```python
from build123d import *

# Parameters (mm, degrees)
SKETCH1_W           = 60
SKETCH1_H           = 52
SKETCH1_R           = 2.9
SKETCH1_R_2         = 3.05
BOSS_EXTRUDE1_DEPTH = 35
SKETCH2_R           = 5.5
CUT_EXTRUDE1_DEPTH  = 7
CHAMFER1_SIZE       = 0.4


with BuildPart() as part:
    # Sketch1 → Boss-Extrude1 (new body)
    with BuildSketch(Plane(origin=(0, 0, 0), x_dir=(1, 0, 0), z_dir=(0, 1, 0))):
        Rectangle(SKETCH1_W, SKETCH1_H)
        with Locations((-23, 6.5)):
            Circle(SKETCH1_R, mode=Mode.SUBTRACT)
        with Locations((23, 6.5)):
            Circle(SKETCH1_R, mode=Mode.SUBTRACT)
        with Locations((23, -6.5)):
            Circle(SKETCH1_R, mode=Mode.SUBTRACT)
        with Locations((-23, -6.5)):
            Circle(SKETCH1_R, mode=Mode.SUBTRACT)
        with Locations((-15, 18.5)):
            Circle(SKETCH1_R_2, mode=Mode.SUBTRACT)
        with Locations((15, 18.5)):
            Circle(SKETCH1_R_2, mode=Mode.SUBTRACT)
        with Locations((15, -18.5)):
            Circle(SKETCH1_R_2, mode=Mode.SUBTRACT)
        with Locations((-15, -18.5)):
            Circle(SKETCH1_R_2, mode=Mode.SUBTRACT)
    extrude(amount=BOSS_EXTRUDE1_DEPTH)

    # Sketch2 → Cut-Extrude1 (cut)
    with BuildSketch(Plane(origin=(0, 35, 0), x_dir=(1, 0, 0), z_dir=(0, 1, 0))):
        with Locations((-15, 18.5)):
            Circle(SKETCH2_R)
        with Locations((15, 18.5)):
            Circle(SKETCH2_R)
        with Locations((15, -18.5)):
            Circle(SKETCH2_R)
        with Locations((-15, -18.5)):
            Circle(SKETCH2_R)
    extrude(amount=-CUT_EXTRUDE1_DEPTH, mode=Mode.SUBTRACT)

    # Chamfer1
    chamfer1_edges = [part.edges().sort_by_distance(p)[0] for p in [
        (-25.9, 35, -6.5),
        (30, 35, 0),
        (20.1, 35, -6.5),
        (0, 35, -26),
        (20.1, 35, 6.5),
        (-25.9, 35, 6.5),
        (-30, 35, 0),
        (0, 0, -26),
        (-20.5, 35, 18.5),
        (30, 0, 0),
        (9.5, 35, 18.5),
        (9.5, 35, -18.5),
        (0, 0, 26),
        (-20.5, 35, -18.5),
        (-30, 0, 0),
        (-30, 17.5, -26),
        (30, 17.5, -26),
        (30, 17.5, 26),
        (-30, 17.5, 26),
        (0, 35, 26),
    ]]
    chamfer(chamfer1_edges, length=CHAMFER1_SIZE)


solid = part.part
```
Input: part model. Units: mm. Frame: model coordinates. A direction names the side the tool comes from. Coordinates: 2 decimals unless noted, no trailing zeros. Loops run counter-clockwise (first coordinate to the right, second up) from the corner with the lowest first, then second, coordinate; pieces in that order, holes last. Notation, with made-up numbers: (64, -24) - (99, -24) arc R6 ccw to (99, -20) - close; hole circle Ø2 at (83, 9). An arc over 180 degrees is marked (long way). Answer in a Markdown table with one row per item.
(1) Set-up query: faces 1 (the face through (-13.36, 13.8, 15.93)), 2 (the face through (-13, 28, -16)). Return all of +Z, -Z, +X, -X, +Y, -Y with unobstructed straight access to the full face (end or side cutting, diameter ignored); none if empty.
Model answer:
| item | result |
|---|---|
| face 1 | +Y, -Y |
| face 2 | +Y |
(2) Cut plane C-C on z = -6.5. Output: boundary loops of the cut face in (x, y), plus the area to 3 significant figures.
Model answer:
| item | result |
|---|---|
| outline | (-30, 0.4) - (-29.6, 0) - (-25.9, 0) - (-25.9, 34.6) - (-26.3, 35) - (-29.6, 35) - (-30, 34.6) - close; (-20.1, 0) - (20.1, 0) - (20.1, 34.6) - (19.7, 35) - (-19.7, 35) - (-20.1, 34.6) - close; (25.9, 0) - (29.6, 0) - (30, 0.4) - (30, 34.6) - (29.6, 35) - (26.3, 35) - (25.9, 34.6) - close |
| area | 1,690 mm² |
(3) Pin query (flat end, axial travel): P1, Ø6.5, axis at x = 15, z = 18.5, coming from the +Y side. Return the tip coordinate at first contact, or that it passes through.
Model answer:
| item | result |
|---|---|
| P1 | stops at y = 28 |
(4) Cut plane A-A on x = -23. Output: boundary loops of the cut face in (y, z), plus the area to 3 significant figures.
Model answer:
| item | result |
|---|---|
| outline | (0, -25.6) - (0.4, -26) - (34.6, -26) - (35, -25.6) - (35, -9.8) - (34.6, -9.4) - (0, -9.4) - close; (0, -3.6) - (34.6, -3.6) - (35, -3.2) - (35, 3.2) - (34.6, 3.6) - (0, 3.6) - close; (0, 9.4) - (34.6, 9.4) - (35, 9.8) - (35, 25.6) - (34.6, 26) - (0.4, 26) - (0, 25.6) - close |
| area | 1,410 mm² |
(5) Cut plane D-D on x = 15. Output: boundary loops of the cut face in (y, z).
Model answer:
| item | result |
|---|---|
| outline | (0, -25.6) - (0.4, -26) - (34.6, -26) - (35, -25.6) - (35, -24.4) - (34.6, -24) - (28, -24) - (28, -21.55) - (0, -21.55) - close; (0, -15.45) - (28, -15.45) - (28, -13) - (34.6, -13) - (35, -12.6) - (35, 12.6) - (34.6, 13) - (28, 13) - (28, 15.45) - (0, 15.45) - close; (0, 21.55) - (28, 21.55) - (28, 24) - (34.6, 24) - (35, 24.4) - (35, 25.6) - (34.6, 26) - (0.4, 26) - (0, 25.6) - close |
(6) Cut plane B-B on y = 19.5. Count the separate pieces of the cut face and the enclosed holes in it, plus the area to 3 significant figures.
Model answer:
| item | result |
|---|---|
| separate pieces | 1 |
| enclosed holes | 8 |
| area | 2,900 mm² |
(7) Mould query, pull axis Z, two halves, no side actions, for faces 3 (the face through (0, 35, 0)), 4 (the face through (20.1, 17.1, -6.6)), 5 (the face through (0, 17, -26)). Classes: pulls with the +Z half, pulls with the -Z half, needs draft (parallel to the pull), parting line crosses it, or undercut.
Model answer:
| item | result |
|---|---|
| face 3 | needs draft |
| face 4 | undercut |
| face 5 | pulls with the -Z half |
(8) Material intervals for L1, parallel to X at y = 29.75, z = 18.5; L2, parallel to Z at x = -23, y = 26; L3, parallel to Z at x = -15, y = 13.75, sorted ascending. Write a range as from..to.
Model answer:
| item | result |
|---|---|
| L1 | x = -30..-20.5, -9.5..9.5, 20.5..30 |
| L2 | z = -26..-9.4, -3.6..3.6, 9.4..26 |
| L3 | z = -26..-21.55, -15.45..15.45, 21.55..26 |
